Design review of the part shown in the three views and the two pictorial views. Dimensions are in mm from the part's minimum x, y and z. Coordinates: 2 decimals unless noted, no trailing zeros. Loops run counter-clockwise (first coordinate to the right, second up) from the corner with the lowest first, then second, coordinate; pieces in that order, holes last. Notation, with made-up numbers: M -31.75,-11.5 L -20.75,-11.5 A23 cw -20.75,3.5 Z; hole C 70,81.25 d11. An arc over 180 degrees is marked long. Answer as a JSON object with one key per item and string values. Group by question number.
Item 1: Wall thickness on L1, parallel to Z at x = 11, y = 1.35; L2, parallel to X at y = 1.05, z = 22.5; L3, parallel to X at y = 0.25, z = 20.5: over which ranges is each line inside the solid? List them lowest first. Write a range as from..to.
Item 2: Add section A-A (x = 31.5). State the section outline as (y, z) points (1 decimal).
Item 3: Add section C-C (x = 23.5). State the section outline as (y, z) points.
Item 4: Insertion check: pin 1 (0.6 mm diameter, centred on x = 17, y = 0.5, fed in from +Z); pin 2 (0.6 mm diameter, centred on y = 1.5, z = 1, fed in from -X). Each pin has a flat end and moves straight along its axis. Give the tip position at first contact, or say it passes through.
Item 5: Add section B-B (y = 0.5). State the section outline as (x, z) points.
Item 6: Add section D-D (z = 6). State the section outline as (x, y) points.
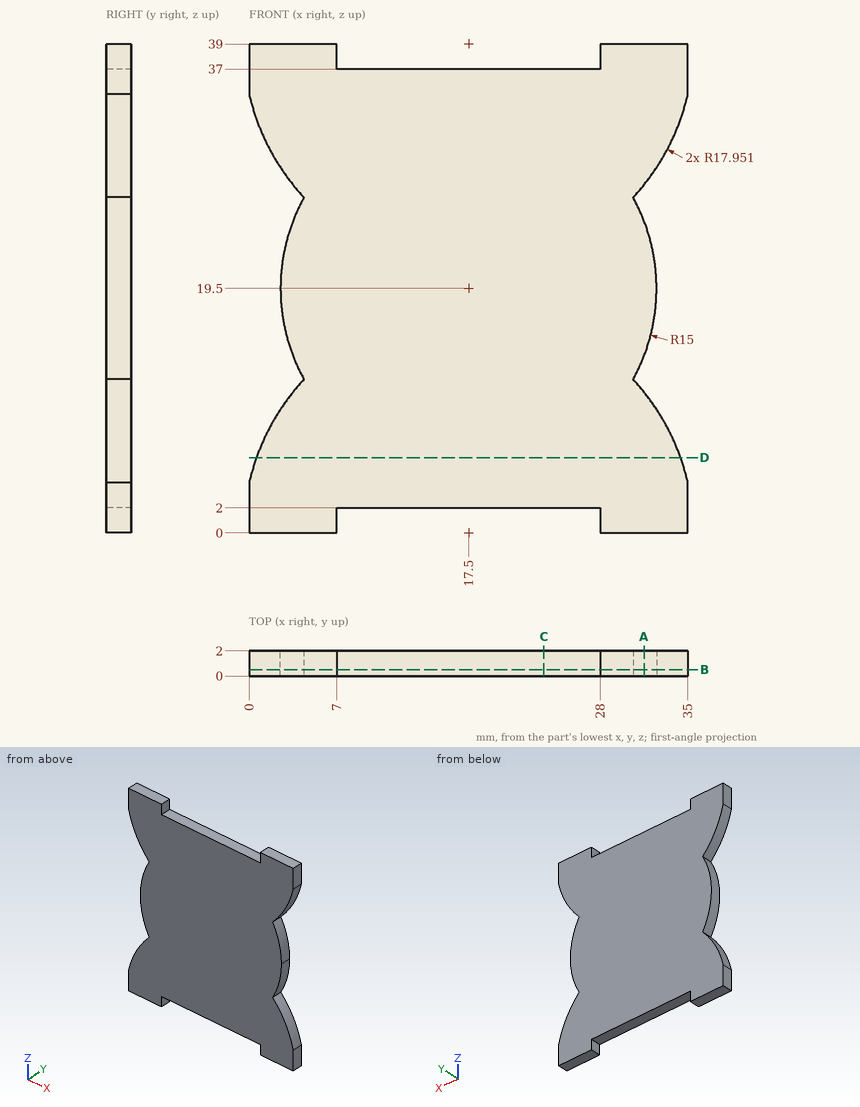
From the geometry:
{
 "1": {"L1": "z = 2..37", "L2": "x = 2.8..32.2", "L3": "x = 2.53..32.47"},
 "2": {"outline": "M 0,0 L 2,0 L 2,11.2 L 0,11.2 Z; M 0,14.1 L 2,14.1 L 2,24.9 L 0,24.9 Z; M 0,27.8 L 2,27.8 L 2,39 L 0,39 Z"},
 "3": {"outline": "M 0,2 L 2,2 L 2,37 L 0,37 Z"},
 "4": {"pin 1": "stops at z = 37", "pin 2": "stops at x = 0"},
 "5": {"outline": "M 0,0 L 7,0 L 7,2 L 28,2 L 28,0 L 35,0 L 35,4 A17.95 ccw 30.63,12.24 A15 ccw 30.63,26.76 A17.95 ccw 35,35 L 35,39 L 28,39 L 28,37 L 7,37 L 7,39 L 0,39 L 0,35 A17.95 ccw 4.37,26.76 A15 ccw 4.37,12.24 A17.95 ccw 0,4 Z"},
 "6": {"outline": "M 0.58,0 L 34.42,0 L 34.42,2 L 0.58,2 Z"}
}
